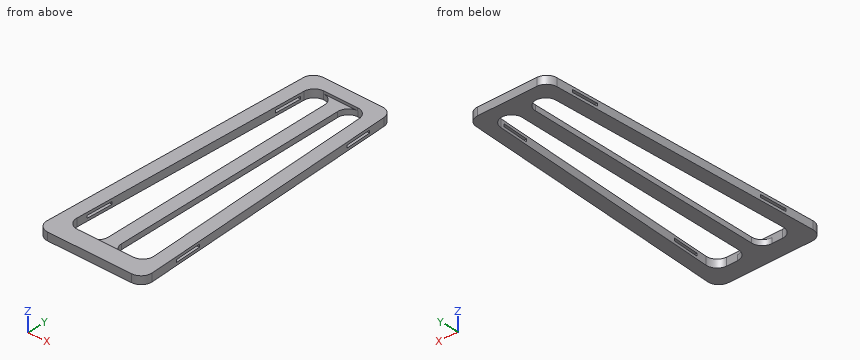
from build123d import *

# Parameters (mm, degrees)
F1_DEPTH = 3.81
F0_W     = 6.35
F0_H     = 124.968
F2_DEPTH = 2.54
F3_W     = 12.7
F3_H     = 1.27
F4_DEPTH = 6.35
F5_W     = 12.7
F5_H     = 1.27
F6_DEPTH = 6.35
F7_F1_R  = 5.08
F7_F2_R  = 5.08
F7_F3_R  = 5.08
F7_F4_R  = 5.08
F7_F5_R  = 5.08
F7_F6_R  = 5.08
F7_F7_R  = 5.08
F7_F8_R  = 5.08
F7_F9_R  = 5.08
F7_F10_R = 5.08
F7_F11_R = 5.08
F7_F12_R = 5.08


with BuildPart() as f1:
    # F0 (on Top) → F1 (new body)
    with BuildSketch(Plane.XY):
        Polygon((6.35, 139.7), (0, 0), (50.8, 0), (44.45, 139.7), align=None)
        Polygon((38.3820798312, 133.35), (44.0624434675, 8.382), (28.575, 8.382), (22.225, 8.382), (6.7375565325, 8.382), (12.4179201688, 133.35), (22.225, 133.35), (28.575, 133.35), align=None, mode=Mode.SUBTRACT)
    extrude(amount=F1_DEPTH)

    # F0 (on Top) → F2 (join)
    with BuildSketch(Plane.XY):
        with Locations((25.4, 70.866)):
            Rectangle(F0_W, F0_H)
    extrude(amount=F2_DEPTH)

    # F3 (on face) → F4 (cut)
    with BuildSketch(Plane(origin=(0, 0, 0), x_dir=(-0.0454076609, -0.9989685402, 0), z_dir=(-0.9989685402, 0.0454076609, 0))):
        with Locations((-120.7942437142, 1.905)):
            Rectangle(F3_W, F3_H)
        with Locations((-25.4, 1.905)):
            Rectangle(F3_W, F3_H)
    extrude(amount=-F4_DEPTH, mode=Mode.SUBTRACT)

    # F5 (on face) → F6 (cut)
    with BuildSketch(Plane(origin=(50.695257732, 2.3043298969, 0), x_dir=(-0.0454076609, 0.9989685402, 0), z_dir=(0.9989685402, 0.0454076609, 0))):
        with Locations((23.0932908253, 1.905)):
            Rectangle(F5_W, F5_H)
        with Locations((118.4875345395, 1.905)):
            Rectangle(F5_W, F5_H)
    extrude(amount=-F6_DEPTH, mode=Mode.SUBTRACT)

    # F7: fillet of radius 5.08 on 12 edges, made by hand

    # F7_f1
    f7_f1_edges = [f1.edges().sort_by_distance(p)[0] for p in [
        (28.575, 8.382, 1.27),
    ]]
    fillet(f7_f1_edges, radius=F7_F1_R)

    # F7_f2
    f7_f2_edges = [f1.edges().sort_by_distance(p)[0] for p in [
        (22.225, 8.382, 1.27),
    ]]
    fillet(f7_f2_edges, radius=F7_F2_R)

    # F7_f3
    f7_f3_edges = [f1.edges().sort_by_distance(p)[0] for p in [
        (28.575, 133.35, 1.27),
    ]]
    fillet(f7_f3_edges, radius=F7_F3_R)

    # F7_f4
    f7_f4_edges = [f1.edges().sort_by_distance(p)[0] for p in [
        (22.225, 133.35, 1.27),
    ]]
    fillet(f7_f4_edges, radius=F7_F4_R)

    # F7_f5
    f7_f5_edges = [f1.edges().sort_by_distance(p)[0] for p in [
        (6.35, 139.7, 1.905),
    ]]
    fillet(f7_f5_edges, radius=F7_F5_R)

    # F7_f6
    f7_f6_edges = [f1.edges().sort_by_distance(p)[0] for p in [
        (0, 0, 1.905),
    ]]
    fillet(f7_f6_edges, radius=F7_F6_R)

    # F7_f7
    f7_f7_edges = [f1.edges().sort_by_distance(p)[0] for p in [
        (44.45, 139.7, 1.905),
    ]]
    fillet(f7_f7_edges, radius=F7_F7_R)

    # F7_f8
    f7_f8_edges = [f1.edges().sort_by_distance(p)[0] for p in [
        (50.8, 0, 1.905),
    ]]
    fillet(f7_f8_edges, radius=F7_F8_R)

    # F7_f9
    f7_f9_edges = [f1.edges().sort_by_distance(p)[0] for p in [
        (38.3820798312, 133.35, 1.905),
    ]]
    fillet(f7_f9_edges, radius=F7_F9_R)

    # F7_f10
    f7_f10_edges = [f1.edges().sort_by_distance(p)[0] for p in [
        (44.0624434675, 8.382, 1.905),
    ]]
    fillet(f7_f10_edges, radius=F7_F10_R)

    # F7_f11
    f7_f11_edges = [f1.edges().sort_by_distance(p)[0] for p in [
        (6.7375565325, 8.382, 1.905),
    ]]
    fillet(f7_f11_edges, radius=F7_F11_R)

    # F7_f12
    f7_f12_edges = [f1.edges().sort_by_distance(p)[0] for p in [
        (12.4179201688, 133.35, 1.905),
    ]]
    fillet(f7_f12_edges, radius=F7_F12_R)


solid = f1.part
Geometry: final body of the model. Coordinates: model frame, mm. Round coordinates to 2 decimals unless told otherwise and drop trailing zeros. Loops run counter-clockwise (first coordinate to the right, second up) from the corner with the lowest first, then second, coordinate; pieces in that order, holes last. Notation, with made-up numbers: (58.5, 25) -> (89.5, 25) arc R18 cw to (89.5, 29) -> close; hole circle Ø1 at (-24, 37). An arc over 180 degrees is marked (long way). One line per question, with ' | ' between items. Start each with the question number.
1. Contact query for flat-ended pins moving along their axis: pin 1 (13 mm diameter, centred on x = 29, y = 49.5, fed in from +Z); pin 2 (0.8 mm diameter, centred on y = 73.5, z = 1, fed in from +X); pin 3 (1 mm diameter, centred on y = 42.5, z = 2.5, fed in from +X). Output: stop coordinate, or through.
2. Section B-B on z = 1.95. Count the separate pieces of the cut face and the enclosed holes in it, and give its area (3 significant figures).
3. Line query: line 1 along Z through (x, y) = (5.5, 22); line 2 along X through (y, z) = (45, 1.2) (3 decimals); line 3 along Y through (x, z) = (27.5, 2.85). Output: solid intervals per line, ascending. Write a range as [from, to].
4. Section A-A on x = 30.5. Output: boundary loops of the cut face in (y, z).
5. Section D-D on x = 47. Output: boundary loops of the cut face in (y, z), and give its area (3 significant figures).
6. Section C-C on y = 103.5. Output: boundary loops of the cut face in (x, z) (3 decimals).
Returned:
1) pin 1: stops at z = 2.54 | pin 2: stops at x = 47.48 | pin 3: stops at x = 48.89
2) separate pieces: 3 | enclosed holes: 0 | area: 2,750 mm2
3) line 1: z = [0, 1.27], [2.54, 3.81] | line 2: x = [2.045, 8.402], [22.225, 28.575], [42.398, 48.755] | line 3: y = [0, 8.38], [133.35, 139.7]
4) outline: (0, 0) -> (9.48, 0) -> (9.48, 2.54) -> (8.38, 2.54) -> (8.38, 3.81) -> (0, 3.81) -> close; (132.25, 0) -> (139.7, 0) -> (139.7, 3.81) -> (133.35, 3.81) -> (133.35, 2.54) -> (132.25, 2.54) -> close
5) outline: (0.23, 0) -> (83.6, 0) -> (83.6, 3.81) -> (0.23, 3.81) -> close; hole (18.9, 1.27) -> (31.61, 1.27) -> (31.61, 2.54) -> (18.9, 2.54) -> close | area: 301 mm2
6) outline: (4.705, 0) -> (11.061, 0) -> (11.061, 3.81) -> (4.705, 3.81) -> close; (22.225, 0) -> (28.575, 0) -> (28.575, 2.54) -> (22.225, 2.54) -> close; (39.739, 0) -> (46.095, 0) -> (46.095, 3.81) -> (39.739, 3.81) -> close
